from build123d import *

# Parameters (mm, degrees)
F1_DEPTH = 12.7
F2_DEPTH = 25.4


with BuildPart() as f1:
    # F0 (on Top) → F1 (new body)
    with BuildSketch(Plane.XY):
        Polygon((106.066017, 136.066017), (0, 30), (106.066017, -76.066017), (109.601551, -72.530483), (7.071068, 30), (109.601551, 132.530483), align=None)
    extrude(amount=F1_DEPTH)

    # F0 (on Top) → F2 (join)
    with BuildSketch(Plane.XY):
        Polygon((-10, 0), (0, 0), (0, 22.928932), (0, 30), (0, 37.071068), (0, 60), (-10, 60), align=None)
        Polygon((0, 30), (0, 22.928932), (102.530483, -79.601551), (106.066017, -76.066017), align=None)
        Polygon((0, 37.071068), (0, 30), (106.066017, 136.066017), (102.530483, 139.601551), align=None)
        Polygon((106.066017, 136.066017), (0, 30), (106.066017, -76.066017), (109.601551, -72.530483), (7.071068, 30), (109.601551, 132.530483), align=None)
    extrude(amount=F2_DEPTH)


solid = f1.part
CAD build for the part. Positions are in the model's coordinates, mm. A direction names the side the tool comes from. Round coordinates to 2 decimals unless told otherwise and drop trailing zeros. Order: outer loops, then holes, each group sorted by start corner. A loop starts at its lowest first (then second) coordinate and runs counter-clockwise, first axis right, second up. Notation, with made-up numbers: (-29.5, 49.5) - (-22.5, 49.5) arc R28 cw to (-22.5, 68.5) - close; hole circle Ø7 at (19, 50). An arc over 180 degrees is marked (long way). Return JSON: item names as keys, results as strings.
(1) Tool access for faces 1 (the face through (-5, 0, 13)), 2 (the face through (0, 11, 13)), 3 (the face through (57.62, 80.55, 12.52)), 4 (the face through (0, 48, 13)): list every direction of +Z, -Z, +X, -X, +Y, -Y with a clear straight run to the whole face (end or side of a thin tool).
Answer key:
{"face 1": "+Z, -Z, -X, -Y", "face 2": "+Z, -Z, -Y", "face 3": "+Z, -Z, +X", "face 4": "+Z, -Z, +Y"}
(2) Pull direction X, two halves, no side cores. Call faces 5 (the face through (50.55, -27.62, 12.52)), 6 (the face through (106.017, -76.116, 12.522)), 7 (the face through (-5, 60, 13)): +X half, -X half, draft (parallel to the pull), parting line (faces both ways), or undercut.
Answer key:
{"face 5": "undercut", "face 6": "+X half", "face 7": "draft"}
(3) Wall check: probe 1 along Y at (x, z) = (24, 12); probe 2 along Y at (x, z) = (76.5, 7.75); probe 3 along X at (y, z) = (9, 21.25). Give the ranges that are in metal, low to high. Write a range as from..to.
Answer key:
{"probe 1": "y = -1.07..13.07, 46.93..61.07", "probe 2": "y = -53.57..-39.43, 99.43..113.57", "probe 3": "x = -10..0, 13.93..28.07"}
(4) Cut at B-B (z = 20.5). Give the cut face in (x, y).
Answer key:
{"outline": "(-10, 0) - (0, 0) - (0, 22.93) - (102.53, -79.6) - (109.6, -72.53) - (7.07, 30) - (109.6, 132.53) - (102.53, 139.6) - (0, 37.07) - (0, 60) - (-10, 60) - close"}
(5) Cut at C-C (y = -39.5). Give the cut face in (x, z), then the cut area to 3 significant figures.
Answer key:
{"outline": "(62.43, 0) - (76.57, 0) - (76.57, 25.4) - (62.43, 25.4) - close", "area": "359 mm^2"}
(6) Pin check, flat tips, straight feed: pin 1 Ø3 at (x, z) = (16.5, 14) entering from +Y; pin 2 Ø2 at (y, z) = (3, 7.5) entering from +X; pin 3 Ø8 at (x, z) = (-5, 15.5) entering from +Y. Stop position of each tip, or through.
Answer key:
{"pin 1": "stops at y = 55.07", "pin 2": "stops at x = 35.07", "pin 3": "stops at y = 60"}
(7) Cut at A-A (x = 72). Give the cut face in (y, z).
Answer key:
{"outline": "(-49.07, 0) - (-34.93, 0) - (-34.93, 25.4) - (-49.07, 25.4) - close; (94.93, 0) - (109.07, 0) - (109.07, 25.4) - (94.93, 25.4) - close"}
